```python
from build123d import *

# Parameters (mm, degrees)
F1_DEPTH = 25
F2_DEPTH = 10
F3_DEPTH = 12.5
F4_DEPTH = 20


with BuildPart() as f1:
    # F0 (on Front) → F1 (new body, symmetric)
    with BuildSketch(Plane.XZ):
        Polygon((0, -41.924461), (0, -9.631296), (-17.999999, -9.631296), (-136.603385, -9.631296), (-136.603385, -41.924461), align=None)
    extrude(amount=F1_DEPTH, both=True)

    # F0 (on Front) → F2 (join, symmetric)
    with BuildSketch(Plane.XZ):
        with BuildLine():
            Line((-136.603385, -9.631296), (-17.999999, -9.631296))
            Line((-17.999999, -9.631296), (-17.999999, 24.361512))
            ThreePointArc((-17.999999, 24.361512), (-9.47987, 45.304653), (11.241012, 54.351908))
            add(Edge.make_bspline(
                [(-136.603385, -9.631296), (-91.775244, 38.556366), (-37.152971, 53.664777), (11.241012, 54.351908)],
                knots=[0, 0, 0, 0, 160.954295, 160.954295, 160.954295, 160.954295], degree=3))
        make_face()
    extrude(amount=F2_DEPTH, both=True)

    # F0 (on Front) → F3 (join, symmetric)
    with BuildSketch(Plane.XZ):
        with BuildLine():
            Line((-17.999999, -9.631296), (0, -9.631296))
            Line((0, -9.631296), (0, 24.361512))
            ThreePointArc((0, 24.361512), (3.514719, 32.846793), (12, 36.361512))
            Line((12, 36.361512), (36.226183, 36.361512))
            Line((36.226183, 36.361512), (36.226183, 54.361511))
            Line((36.226183, 54.361511), (12, 54.361511))
            add(Edge.make_bspline(
                [(11.241012, 54.351908), (11.494179, 54.355503), (11.747176, 54.358703), (12, 54.361511)],
                knots=[160.954295, 160.954295, 160.954295, 160.954295, 161.796308, 161.796308, 161.796308, 161.796308], degree=3))
            ThreePointArc((11.241012, 54.351908), (-9.47987, 45.304653), (-17.999999, 24.361512))
            Line((-17.999999, 24.361512), (-17.999999, -9.631296))
        make_face()
    extrude(amount=F3_DEPTH, both=True)

    # F0 (on Front) → F4 (join, symmetric)
    with BuildSketch(Plane.XZ):
        Polygon((36.226183, 54.361511), (36.226183, 36.361512), (36.226183, 26.344426), (90.614673, 26.344426), (90.614673, 61.187055), (36.226183, 61.187055), align=None)
    extrude(amount=F4_DEPTH, both=True)


solid = f1.part
```
The listing builds one solid part. Answer for the finished solid, in the listing's coordinates (mm). A direction names the side the tool comes from. Round coordinates to 2 decimals unless told otherwise and drop trailing zeros. Write each loop counter-clockwise with the first axis right and the second up, starting at its lowest first coordinate (ties: lowest second). Pieces come first, ordered by that corner, then holes. Notation, with made-up numbers: (55, 65) -> (70, 65) arc R32 cw to (70, 94) -> close; hole circle Ø8 at (23.25, 43.25). An arc over 180 degrees is marked (long way). Use CSV: the item, a comma, the result in double quotes. Start each with the question number.
(1) Each of these flat-tipped pins is pushed along its axis until it touches: pin 1 (7.5 mm diameter, centred on x = 21, y = 4.5, fed in from +Z); pin 2 (0.8 mm diameter, centred on y = -11, z = 10.5, fed in from -X); pin 3 (3 mm diameter, centred on y = 12, z = -25, fed in from +X). Where does it stop, or does it pass through?
(2) Section A-A on x = 43 is taken. Give the vertices of the cut face in (y, z).
(3) Consider L1, parallel to X at y = -15, z = 40; L2, parallel to X at y = -7.5, z = -30.5; L3, parallel to Z at x = -63, y = -23. Determine where each line is inside the solid, lowest interval first. Write a range as from..to.
(4) Section B-B on z = -27 is taken. Give the vertices of the cut face in (x, y), then the cut area to 3 significant figures.
(5) Which of the six approach directions +Z, -Z, +X, -X, +Y, -Y give full straight-line access (tool end or side, diameter ignored) to faces 1 (the face through (63, 0, 26.344)), 2 (the face through (24, 0, 54.362)), 3 (the face through (-9.25, 11.23, 45.54))?
A:
1,pin 1,"stops at z = 54.36"
1,pin 2,"stops at x = -18"
1,pin 3,"stops at x = 0"
2,outline,"(-20, 26.34) -> (20, 26.34) -> (20, 61.19) -> (-20, 61.19) -> close"
3,L1,"x = 36.23..90.61"
3,L2,"x = -136.6..0"
3,L3,"z = -41.92..-9.63"
4,outline,"(-136.6, -25) -> (0, -25) -> (0, 25) -> (-136.6, 25) -> close"
4,area,"6,830 mm²"
5,face 1,"-Z, +X, +Y, -Y"
5,face 2,"+Z, -X, +Y, -Y"
5,face 3,"+Z, -X, +Y"
